Design review of the part shown in the three views and the two pictorial views. Dimensions are in mm from the part's minimum x, y and z. A direction names the side the tool comes from. Coordinates: 2 decimals unless noted, no trailing zeros. Loops run counter-clockwise (first coordinate to the right, second up) from the corner with the lowest first, then second, coordinate; pieces in that order, holes last. Notation, with made-up numbers: M 84,-13 L 111,-13 A21 ccw 111,11 Z; hole C -28,12 d6. An arc over 180 degrees is marked long. Answer as a JSON object with one key per item and string values. Group by question number.
Item 1: Add section A-A (z = 7.5). State the section outline as (x, y) points.
Item 2: Insertion check: pin 1 (4 mm diameter, centred on x = 6, y = 4.5, fed in from -Z). The pin has a flat end and moves straight along its axis. Give the tip position at first contact, or say it passes through.
Item 3: Mouldability with a two-part tool opening along X and no side actions: class the marked faces 3, 4 and 5 as +X half, -X half, draft (parallel to the pull), parting line (faces both ways), or undercut.
Item 4: Add section C-C (x = 5). State the section outline as (y, z) points.
Item 5: Add section B-B (y = 25). State the section outline as (x, z) points.
Item 6: Tool access review of the marked faces 1 and 2: name each direction out of +Z, -Z, +X, -X, +Y, -Y from which nothing blocks a thin tool from reaching the whole face with its end or side.
Item 7: Wall thickness on L1, parallel to Y at x = 5, z = 4.75; L2, parallel to Y at x = 4, z = 2.5; L3, parallel to Z at x = 2.5, y = 13: over which ranges is each line inside the solid? List them lowest first. Write a range as from..to.
Item 8: Add section D-D (y = 15). State the section outline as (x, z) points.
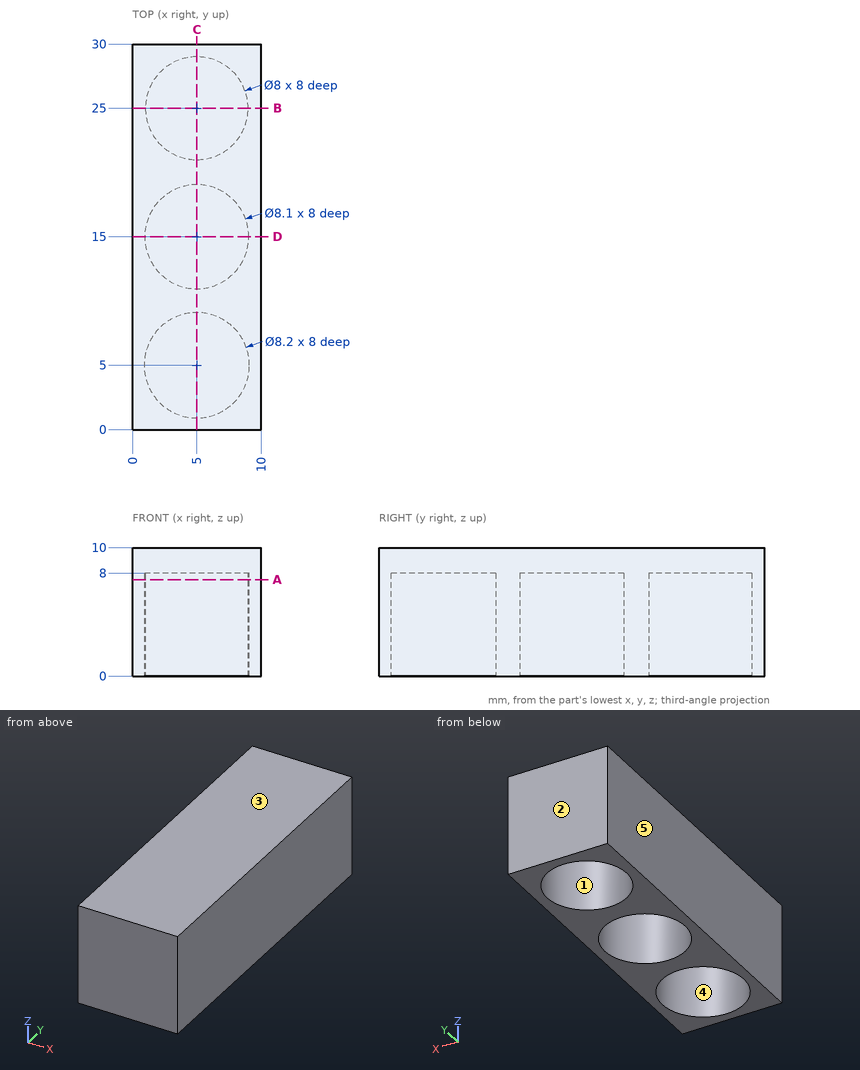
From the geometry:
{
 "1": {"outline": "M 0,0 L 10,0 L 10,30 L 0,30 Z; hole C 5,5 d8.2; hole C 5,15 d8.1; hole C 5,25 d8"},
 "2": {"pin 1": "stops at z = 8"},
 "3": {"face 3": "draft", "face 4": "undercut", "face 5": "-X half"},
 "4": {"outline": "M 0,0 L 0.9,0 L 0.9,8 L 9.1,8 L 9.1,0 L 10.95,0 L 10.95,8 L 19.05,8 L 19.05,0 L 21,0 L 21,8 L 29,8 L 29,0 L 30,0 L 30,10 L 0,10 Z"},
 "5": {"outline": "M 0,0 L 1,0 L 1,8 L 9,8 L 9,0 L 10,0 L 10,10 L 0,10 Z"},
 "6": {"face 1": "-Z", "face 2": "+Z, -Z, +X, -X, +Y"},
 "7": {"L1": "y = 0..0.9, 9.1..10.95, 19.05..21, 29..30", "L2": "y = 0..1.02, 8.98..11.08, 18.92..21.13, 28.87..30", "L3": "z = 8..10"},
 "8": {"outline": "M 0,0 L 0.95,0 L 0.95,8 L 9.05,8 L 9.05,0 L 10,0 L 10,10 L 0,10 Z"}
}
